The listing builds one solid part. Answer for the finished solid, in the listing's coordinates (mm). Round coordinates to 2 decimals unless told otherwise and drop trailing zeros. Loops run counter-clockwise (first coordinate to the right, second up) from the corner with the lowest first, then second, coordinate; pieces in that order, holes last. Notation, with made-up numbers: (63, 15.25) - (97, 15.25) arc R21 cw to (97, 40.25) - close; hole circle Ø6 at (86.5, 49). An arc over 180 degrees is marked (long way). Write item = value, one per line. Start each with the question number.
1) Section B-B, the plane z = 7 is taken. Determine the outline of the cut face in (x, y), and give its area (3 significant figures).
2) For a pull along Y with two mould halves and no side action, classify faces 1 (the cylindrical face through (-7.215, -11.846, 7.199)), 2 (the flat face through (0, 15, 4)), 3 (the flat face through (0, -15, 4)), 4 (the cylindrical face through (-4, 0, 4)) as released by +Y, released by -Y, zero draft, split by the parting line, or undercut.
3) Section A-A, the plane z = 5.75 is taken. Determine the outline of the cut face in (x, y).
4) Straight lines are drawn through the part: line 1 along Y through (x, z) = (6.5, 5.25); line 2 along Y through (x, z) = (7.25, 2.25); line 3 along X through (y, z) = (-8.5, 4.75). For each, find the intervals that lie inside material, in ascending order.
from build123d import *

# Parameters (mm, degrees)
PAD_DEPTH    = 7.5
SKETCH001_R  = 14
POCKET_DEPTH = 7.501
FILLET_R     = 1


with BuildPart() as part:
    # Sketch → Pad (new body)
    with BuildSketch(Plane.XY):
        Polygon((0, 15), (-7.5, 15), (-7.5, 0), (-7.5, -15), (0, -15), (7.5, -15), (7.5, 0), (7.5, 15), align=None)
    extrude(amount=PAD_DEPTH)

    # Sketch001 → Pocket (cut, through all)
    with BuildSketch(Plane(origin=(0, 0, 0), x_dir=(1, 0, 0), z_dir=(0, 0, -1))):
        with Locations((18, 0)):
            Circle(SKETCH001_R)
        with Locations((-18, 0)):
            Circle(SKETCH001_R)
    extrude(amount=-POCKET_DEPTH, mode=Mode.SUBTRACT)

    # Fillet
    fillet_edges = [part.edges().sort_by_distance(p)[0] for p in [
        (-7.5, -12.130065, 7.5),
        (-3.75, -15, 7.5),
        (3.75, -15, 7.5),
        (7.5, -12.130065, 7.5),
        (-7.5, -12.130065, 0),
        (-7.5, -15, 3.75),
        (-7.5, -9.26013, 3.75),
        (-4.904199, -4.949747, 7.5),
        (-4.904199, 4.949747, 7.5),
        (-4.904199, 4.949747, 0),
        (-4.904199, -4.949747, 0),
        (-7.5, 9.26013, 3.75),
        (-7.5, 12.130065, 0),
        (-7.5, 12.130065, 7.5),
        (-7.5, 15, 3.75),
        (-3.75, 15, 7.5),
        (3.75, 15, 7.5),
        (7.5, 12.130065, 7.5),
        (4, 0, 7.5),
        (7.5, -15, 3.75),
        (7.5, -12.130065, 0),
        (4, 0, 0),
        (7.5, 12.130065, 0),
        (7.5, 9.26013, 3.75),
        (7.5, -9.26013, 3.75),
        (7.5, 15, 3.75),
        (-3.75, 15, 0),
        (3.75, 15, 0),
        (-3.75, -15, 0),
        (3.75, -15, 0),
    ]]
    fillet(fillet_edges, radius=FILLET_R)


solid = part.part
Geometry check:
q1.outline = (-7.37, -14) arc R0.87 ccw to (-6.5, -14.87) - (6.5, -14.87) arc R0.87 ccw to (7.37, -14) - (7.37, -9.63) arc R0.87 ccw to (7.16, -9.07) arc R14.13 cw to (7.16, 9.07) arc R0.87 ccw to (7.37, 9.63) - (7.37, 14) arc R0.87 ccw to (6.5, 14.87) - (-6.5, 14.87) arc R0.87 ccw to (-7.37, 14) - (-7.37, 9.63) arc R0.87 ccw to (-7.16, 9.07) arc R14.13 cw to (-7.16, -9.07) arc R0.87 ccw to (-7.37, -9.63) - close
q1.area = 348 mm2
q2.face_1 = zero draft
q2.face_2 = released by +Y
q2.face_3 = released by -Y
q2.face_4 = undercut
q3.outline = (-7.5, -14) arc R1 ccw to (-6.5, -15) - (6.5, -15) arc R1 ccw to (7.5, -14) - (7.5, -9.63) arc R1 ccw to (7.27, -8.99) arc R14 cw to (7.27, 8.99) arc R1 ccw to (7.5, 9.63) - (7.5, 14) arc R1 ccw to (6.5, 15) - (-6.5, 15) arc R1 ccw to (-7.5, 14) - (-7.5, 9.63) arc R1 ccw to (-7.27, 8.99) arc R14 cw to (-7.27, -8.99) arc R1 ccw to (-7.5, -9.63) - close
q4.line_1 = -15 to -7.98, 7.98 to 15
q4.line_2 = -14.66 to -8.97, 8.97 to 14.66
q4.line_3 = -6.88 to 6.88
